```python
from build123d import *

# Parameters (mm, degrees)
F1_R     = 51.4012769419
F1_R_2   = 42.5693345022
F2_DEPTH = 9
F3_DEPTH = 58.5
F4_DEPTH = 4.15
F5_W     = 153.4909196198
F5_H     = 81.327278167
F6_DEPTH = 9
F7_DEPTH = 81.9
F8_DEPTH = 2.2


with BuildPart() as f2:
    # F1 (on Top) → F2 (new body)
    with BuildSketch(Plane.XY):
        with Locations((92.0659080148, 0)):
            Circle(F1_R)
        with Locations((92.0659080148, 0)):
            Circle(F1_R_2, mode=Mode.SUBTRACT)
    extrude(amount=-F2_DEPTH)

    # F1 (on Top) → F3 (join)
    with BuildSketch(Plane.XY):
        with Locations((92.0659080148, 0)):
            Circle(F1_R)
        with Locations((92.0659080148, 0)):
            Circle(F1_R_2, mode=Mode.SUBTRACT)
    extrude(amount=F3_DEPTH)

    # F0 (on Front) → F4 (join, symmetric)
    with BuildSketch(Plane.XZ):
        Polygon((55.6977316737, 45.6750020385), (-64.4393563271, -11.1907897517), (55.6977316737, -11.1907897517), align=None)
    extrude(amount=F4_DEPTH, both=True)

    # F5 (on Top) → F6 (join)
    with BuildSketch(Plane.XY):
        with Locations((-15.1641424745, 1.2886393815)):
            Rectangle(F5_W, F5_H)
    extrude(amount=-F6_DEPTH)

    # F7 (cut): faces of the model
    f7_faces = [f2.faces().sort_by_distance(p)[0] for p in [
        (57.1486967717, 0, 0),
        (52.6306177028, 0, 44.2232116932),
    ]]
    extrude(f7_faces, amount=-F7_DEPTH, dir=(0, 0, 1), mode=Mode.SUBTRACT)

    # F8 (cut): a face of the model
    f8_faces = [f2.faces().sort_by_distance(p)[0] for p in [
        (-7.4376125562, 1e-10, -11.1907897517),
    ]]
    extrude(f8_faces, amount=-F8_DEPTH, mode=Mode.SUBTRACT)


solid = f2.part
```
The model under review builds one solid part; all positions refer to its coordinate system, in mm. A direction names the side the tool comes from. Round coordinates to 2 decimals unless told otherwise and drop trailing zeros. Order: outer loops, then holes, each group sorted by start corner. A loop starts at its lowest first (then second) coordinate and runs counter-clockwise, first axis right, second up. Notation, with made-up numbers: (75, 31) -> (117, 31) arc R30 cw to (117, 57) -> close; hole circle Ø8 at (-23.5, -19.5). An arc over 180 degrees is marked (long way). One line per item, written item: value. Start each with the question number.
Q1. Machinability: for faces 1 (the face through (18, 4.15, 11)), 2 (the face through (-17, -39.375, -4)), 3 (the face through (-16, 11, 0)), 4 (the face through (18, -4.15, 11)), 5 (the face through (-16, 41.952, -4)), which of the approach directions +Z, -Z, +X, -X, +Y, -Y give a long, thin tool a straight path to every point of the face, cutting with its end or side? Answer none if there is none.
Q2. Wall thickness on line 1 (X direction, y = -2, z = 50.5); line 2 (X direction, y = 0, z = 20); line 3 (Y direction, x = 128.5, z = 53.5): over which ranges is each line inside the solid? List them lowest first.
Q3. Take a section at B-B (x = 85). Write out the cut boundary in (y, z).
Q4. Take a section at D-D (z = 48). Write out the cut boundary in (x, y), and give its area (3 significant figures).
Q5. Take a section at A-A (y = -15). Write out the cut boundary in (x, z).
Q6. Clearance check with flat-ended pins moving along their axes: pin 1 Ø10 at (x, z) = (-32, -2.5) entering from -Y (3 decimals); pin 2 Ø1 at (x, z) = (23, 10) entering from -Y; pin 3 Ø6 at (x, z) = (31, 8) entering from +Y. State where each tip first meets the part, or that it passes through.
Q7. Take a section at C-C (x = -45). Write out the cut boundary in (y, z) (3 decimals).
Reported:
1. face 1: +Z, -X, +Y
1. face 2: +Z, -Z, -X, -Y
1. face 3: +Z, -X
1. face 4: +Z, -X, -Y
1. face 5: +Z, -Z, -X, +Y
2. line 1: x = 40.7 to 49.54, 134.59 to 143.43
2. line 2: x = 1.46 to 49.5, 134.64 to 143.47
2. line 3: y = -36.26 to -22.02, 22.02 to 36.26
3. outline: (-50.91, -9) -> (-41.98, -9) -> (-41.98, 58.5) -> (-50.91, 58.5) -> close; (41.98, -9) -> (50.91, -9) -> (50.91, 58.5) -> (41.98, 58.5) -> close
4. outline: circle Ø102.8 at (92.07, 0); hole circle Ø85.14 at (92.07, 0)
4. area: 2,610 mm2
5. outline: (-91.91, -9) -> (52.23, -9) -> (52.23, 58.5) -> (42.9, 58.5) -> (42.9, 0) -> (-91.91, 0) -> close; (131.9, -9) -> (141.23, -9) -> (141.23, 58.5) -> (131.9, 58.5) -> close
6. pin 1: stops at y = -39.375
6. pin 2: stops at y = -4.15
6. pin 3: stops at y = 4.15
7. outline: (-39.375, -9) -> (-4.15, -9) -> (-4.15, -8.991) -> (4.15, -8.991) -> (4.15, -9) -> (41.952, -9) -> (41.952, 0) -> (-39.375, 0) -> close
